from build123d import *

# Parameters (mm, degrees)
F0_W         = 78.1229734421
F0_H         = 58.4978777915
F1_DEPTH     = 48.514
F2_R         = 5.08
F3_T1_DEPTH  = 67.9629734421
F3_S5_W      = 5.08
F3_S5_H      = 5.08
F3_T6_DEPTH  = 5.08
F3_S11_W     = 5.08
F3_S11_H     = 5.08
F3_T12_DEPTH = 5.08
F4_T         = -2.54


# Not quite as in the source:
# - a fillet or chamfer that OpenCascade refuses, or shapes differently, is made with other operations: its cross-section is extruded or revolved along the edge and cut away or added
# - a shell that OpenCascade refuses in one call is made with other operations: the cavity is built on its own and cut out


with BuildPart() as f1:
    # F0 (on Top) → F1 (new body)
    with BuildSketch(Plane.XY):
        with Locations((-6.4158961177, 8.1142215058)):
            Rectangle(F0_W, F0_H)
    extrude(amount=F1_DEPTH)

    # F2
    f2_edges = [f1.edges().sort_by_distance(p)[0] for p in [
        (-6.415896, -21.134717, 48.514),
        (-45.477383, 8.114222, 48.514),
        (-6.415896, 37.36316, 48.514),
        (32.645591, 8.114222, 48.514),
        (32.645591, -21.134717, 24.257),
        (32.645591, 8.114222, 0),
        (32.645591, 37.36316, 24.257),
        (-45.477383, -21.134717, 24.257),
        (-45.477383, 37.36316, 24.257),
        (-45.477383, 8.114222, 0),
        (-6.415896, 37.36316, 0),
    ]]
    fillet(f2_edges, radius=F2_R)

    # F3: fillet of radius 5.08 on 1 edges, made by hand

    # F3_s2 → F3_t1 (cut)
    with BuildSketch(Plane.YZ.offset(-40.3973828387)):
        with BuildLine():
            ThreePointArc((-16.0547173899, 0), (-19.6468198384, 1.4878975516), (-21.1347173899, 5.08))
            Line((-21.1347173899, 5.08), (-21.1347173899, 0))
            Line((-21.1347173899, 0), (-16.0547173899, 0))
        make_face()
    extrude(amount=F3_T1_DEPTH, mode=Mode.SUBTRACT)


with BuildPart() as f3_tool4:
    # F3_s5 → F3_t6 (new body)
    with BuildSketch(Plane.XY.offset(5.08)):
        with Locations((-42.9373828387, -18.5947173899)):
            Rectangle(F3_S5_W, F3_S5_H)
    extrude(amount=-F3_T6_DEPTH)

    # F3_s7 → F3_t8 (revolve, cut)
    with BuildSketch(Plane(origin=(-40.3973828387, -16.0547173899, 5.08), x_dir=(0.7071067812, 0.7071067812, 0), z_dir=(-0.7071067812, 0.7071067812, 0))):
        with BuildLine():
            ThreePointArc((0, -5.08), (5.08, 0), (0, 5.08))
            Line((0, 5.08), (0, -5.08))
        make_face()
    revolve(axis=Axis((-40.3973828387, -16.0547173899, 5.08), (0, 0, -1)), mode=Mode.SUBTRACT)


with BuildPart() as f1_1:
    add(f1.part)

    # F3_t3: cut F3_tool4
    add(f3_tool4.part, mode=Mode.SUBTRACT)


with BuildPart() as f3_tool10:
    # F3_s11 → F3_t12 (new body)
    with BuildSketch(Plane.XY.offset(5.08)):
        with Locations((30.1055906034, -18.5947173899)):
            Rectangle(F3_S11_W, F3_S11_H)
    extrude(amount=-F3_T12_DEPTH)

    # F3_s13 → F3_t14 (revolve, cut)
    with BuildSketch(Plane(origin=(27.5655906034, -16.0547173899, 5.08), x_dir=(-0.7071067812, 0.7071067812, 0), z_dir=(-0.7071067812, -0.7071067812, 0))):
        with BuildLine():
            ThreePointArc((0, -5.08), (5.08, 0), (0, 5.08))
            Line((0, 5.08), (0, -5.08))
        make_face()
    revolve(axis=Axis((27.5655906034, -16.0547173899, 5.08), (0, 0, -1)), mode=Mode.SUBTRACT)


with BuildPart() as f1_2:
    add(f1_1.part)

    # F3_t9: cut F3_tool10
    add(f3_tool10.part, mode=Mode.SUBTRACT)

    # F4: a shell. OpenCascade refuses it in one call, so the cavity is built on its own and cut out:
    # the body offset inwards by the wall thickness, plus a prism from it out through each open face.
    f4_core = offset(f1_2.part, amount=F4_T, mode=Mode.PRIVATE)
    f4_exits = [f4_core.faces().sort_by_distance(p)[0] for p in [
        (-6.415896, -18.594717, 24.257),
    ]]
    add(f4_core, mode=Mode.SUBTRACT)
    extrude(f4_exits, amount=-F4_T, mode=Mode.SUBTRACT)


solid = f1_2.part
Check sheet for the modelled part. Datum: model origin and axes. Units: mm. A direction names the side the tool comes from. Round coordinates to 2 decimals unless told otherwise and drop trailing zeros. Order: outer loops, then holes, each group sorted by start corner. A loop starts at its lowest first (then second) coordinate and runs counter-clockwise, first axis right, second up. Notation, with made-up numbers: M 49,36.5 L 85,36.5 A22 ccw 85,57.5 Z; hole C 10.25,28 d10. An arc over 180 degrees is marked long. One line per item, written item: value. Start each with the question number.
1. Gauge pin test, flat ends, axial feed: P1, Ø0.8, axis at y = -19.5, z = 18.5, coming from the -X side; P2, Ø1.3, axis at x = -22.5, y = -19.5, coming from the +Z side; P3, Ø0.8, axis at x = -7.5, y = -20.5, coming from the -Z side. Record the tip position at first contact, or that the pin passes through.
2. Release check for a two-part mould opening along Y. For faces 1 (the flat face through (-7, 8, 45.974)), 2 (the flat face through (30.106, 8, 24)), 3 (the cylindrical face through (31.197, 35.836, 24.525)), 4 (the cylindrical face through (-44, 8.5, 1.5)) record: released by +Y, released by -Y, zero draft, split by the parting line, or undercut.
3. Section check B-B on z = 33. Enter the section's corners in (x, y), and give its area (3 significant figures).
4. Section check C-C on x = -5. Enter the section's corners in (y, z), and give its area (3 significant figures).
5. Access from +Z, -Z, +X, -X, +Y, -Y to the whole of each face (thin tool, end or side, straight path). Record for faces 5 (the cylindrical face through (29.38, 8.45, 45.21)), 6 (the cylindrical face through (-5.94, 35.915, 1.528)), 7 (the flat face through (-7, -20, 43.434)).
6. Section check A-A on y = 27. Enter the section's corners in (x, z).
7. Scan lines: line 1 along Z through (x, y) = (-19.5, -12); line 2 along X through (y, z) = (-2.5, 5); line 3 along Y through (x, z) = (-18, 31.5). Record each from-to range of solid material in increasing order.
Results found:
1. P1: x = -44.46
1. P2: z = 47.68
1. P3: z = 2.01
2. face 1: undercut
2. face 2: undercut
2. face 3: released by +Y
2. face 4: zero draft
3. outline: M -45.48,-16.05 A5.08 ccw -40.4,-21.13 L -40.4,-18.59 A2.54 cw -42.94,-16.05 L -42.94,32.28 A2.54 cw -40.4,34.82 L 27.57,34.82 A2.54 cw 30.11,32.28 L 30.11,-16.05 A2.54 cw 27.57,-18.59 L 27.57,-21.13 A5.08 ccw 32.65,-16.05 L 32.65,32.28 A5.08 ccw 27.57,37.36 L -40.4,37.36 A5.08 ccw -45.48,32.28 Z
3. area: 479 mm^2
4. outline: M -21.13,5.08 A5.08 ccw -16.05,0 L 32.28,0 A5.08 ccw 37.36,5.08 L 37.36,43.43 A5.08 ccw 32.28,48.51 L -16.05,48.51 A5.08 ccw -21.13,43.43 L -18.59,43.43 A2.54 cw -16.05,45.97 L 32.28,45.97 A2.54 cw 34.82,43.43 L 34.82,5.08 A2.54 cw 32.28,2.54 L -16.05,2.54 A2.54 cw -18.59,5.08 Z
4. area: 404 mm^2
5. face 5: none
5. face 6: -Z, +X, -X, +Y
5. face 7: -Y
6. outline: M -45.48,5.08 A5.08 ccw -40.4,0 L 27.57,0 A5.08 ccw 32.65,5.08 L 32.65,43.43 A5.08 ccw 27.57,48.51 L -40.4,48.51 A5.08 ccw -45.48,43.43 Z; hole M -42.94,5.08 A2.54 ccw -40.4,2.54 L 27.57,2.54 A2.54 ccw 30.11,5.08 L 30.11,43.43 A2.54 ccw 27.57,45.97 L -40.4,45.97 A2.54 ccw -42.94,43.43 Z
7. line 1: 0 to 2.54, 45.97 to 48.51
7. line 2: -45.48 to -42.94, 30.1 to 32.64
7. line 3: 34.82 to 37.36
